Could you check a few things on this model? Use its own coordinates, in mm. A direction names the side the tool comes from. Round coordinates to 2 decimals unless told otherwise and drop trailing zeros. Loops run counter-clockwise (first coordinate to the right, second up) from the corner with the lowest first, then second, coordinate; pieces in that order, holes last.
Autodesk Inventor part; units mm, degrees
ref_plane "YZ Plane" through (0, 0, 0) normal (1, 0, 0) x (0, 1, 0)
ref_plane "XZ Plane" through (0, 0, 0) normal (0, 1, 0) x (-1, 0, 0)
ref_plane "XY Plane" through (0, 0, 0) normal (0, 0, 1) x (1, 0, 0)
sketch "スケッチ1" plane through (0, 0, 0) normal (0, 1, 0) x (-1, 0, 0)
  line L0 (0, 0) -> (30, 0)
  line L1 (30, 0) -> (30, -30)
  line L2 (30, -30) -> (0, -30)
  line L3 (0, -30) -> (0, 0)
  circle A0 centre (25, -5) radius 1.5
  circle A1 centre (25, -25) radius 1.5
  circle A2 centre (5, -5) radius 1.5
  circle A3 centre (5, -25) radius 1.5
  dimension "d18" = 30
  dimension "d19" = 30
  dimension "d20" = 3
  dimension "d21" = 3
  dimension "d22" = 20
  dimension "d23" = 5
  dimension "d24" = 5
  dimension "d25" = 3
  dimension "d26" = 3
  dimension "d27" = 20
extrude "押し出し1" add sketch "スケッチ1" along normal blind 5
sketch "スケッチ2" plane through (0, 5, 0) normal (0, 1, 0) x (1, 0, 0)
  circle A0 centre (-15, 15) radius 10
  line L0 (0, 30) -> (-30, 30)
  line L1 (-30, 30) -> (-30, 0)
  point P0 (0, 0)
  dimension "d32" = 20
  dimension "d33" = 15
  dimension "d34" = 15
extrude "押し出し2" add sketch "スケッチ2" along normal blind 12
sketch "スケッチ9" plane through (-15, 17, -15) normal (0, 1, 0) x (1, 0, 0)
  circle A0 centre (0, 0) radius 10
  circle A1 centre (0, 0) radius 10
  point P0 (15, -15)
extrude "押し出し4" add sketch "スケッチ9" along normal blind 10
fillet "フィレット1" radius 10 1 edges at (-25, 27, -15)
properties part number "ballcaster" material "ポリプロピレン"
Item 1: We'd pull the mould along Z, two halves only. Please class faces 1 (the cylindrical face through (-23.89, 2.46, -26.01)), 2 (the flat face through (-4.8, 5, -14.8)), 3 (the flat face through (-15, 2, -30)): released by +Z, released by -Z, zero draft, split by the parting line, or undercut.
Results list:
face 1: undercut
face 2: zero draft
face 3: released by -Z
Item 2: If we section it at A-A, the plane z = -6: Please give me the cut outline in (x, y), then the cut area to 3 significant figures.
Results list:
outline: (-30, 0) - (-26.12, 0) - (-26.12, 5) - (-30, 5) - close; (-23.88, 0) - (-6.12, 0) - (-6.12, 5) - (-10.64, 5) - (-10.64, 17) arc R4.36 ccw to (-19.36, 17) - (-19.36, 5) - (-23.88, 5) - close; (-3.88, 0) - (0, 0) - (0, 5) - (-3.88, 5) - close
area: 262 mm2
Item 3: If we section it at C-C, the plane y = 9.5: Please give me the cut outline in (x, z).
Results list:
outline: circle Ø20 at (-15, -15)
Item 4: If we section it at B-B, the plane x = -15: Please give me the cut outline in (y, z).
Results list:
outline: (0, -30) - (5, -30) - (5, -25) - (17, -25) arc R10 ccw to (17, -5) - (5, -5) - (5, 0) - (0, 0) - close
Item 5: If we section it at D-D, the plane z = -25.75: Please give me the cut outline in (x, y), then the cut area to 3 significant figures.
Results list:
outline: (-30, 0) - (-26.3, 0) - (-26.3, 5) - (-30, 5) - close; (-23.7, 0) - (-6.3, 0) - (-6.3, 5) - (-23.7, 5) - close; (-3.7, 0) - (0, 0) - (0, 5) - (-3.7, 5) - close
area: 124 mm2
Item 6: If I drill on line 1 along Z through (x, y) = (-25, 1.2); line 2 along Y through (x, z) = (-28, -20.5); line 3 along Z through (x, y) = (-14.75, 8.25), over which ranges is the centre line in solid material (lowest first)?
Results list:
line 1: z = -30 to -26.5, -23.5 to -6.5, -3.5 to 0
line 2: y = 0 to 5
line 3: z = -25 to -5
Item 7: For faces 4 (the cylindrical face through (-5.46, 10.92, -12)), 5 (the flat face through (-15, 2, 0)), which set-ups out of +Z, -Z, +X, -X, +Y, -Y let a thin tool reach every point of the face, with its end or its side?
Results list:
face 4: +Y
face 5: +Z, +X, -X, +Y, -Y
Item 8: Will these pins go through, and if not, where does the flat tip stop? pin 1 (4 mm diameter, centred on x = -19, y = 22, fed in from +Z); pin 2 (6 mm diameter, centred on x = -18.5, z = -25, fed in from +Y); pin 3 (1.8 mm diameter, centred on x = -25, z = -25, fed in from +Y); pin 4 (8 mm diameter, centred on x = -10.5, z = -14, fed in from +Y).
Results list:
pin 1: stops at z = -6.02
pin 2: stops at y = 23.51
pin 3: passes through
pin 4: stops at y = 26.98
